from build123d import *

# Parameters (mm, degrees)
SKETCH1_R           = 75
BOSS_EXTRUDE1_DEPTH = 6.35
SKETCH2_W           = 18
SKETCH2_H           = 12
CUT_EXTRUDE1_DEPTH  = 144.69092772
CIRPATTERN1_COUNT   = 20


with BuildPart() as part:
    # Sketch1 → Boss-Extrude1 (new body)
    with BuildSketch(Plane.XY):
        with BuildLine():
            Line((-85.524663655, 39.880805624), (-96.4003571, 44.952224764))
            ThreePointArc((-96.4003571, 44.952224764), (-9.270409947, 105.961270564), (87.129947152, 61.0090458))
            Line((87.129947152, 61.0090458), (77.300122621, 54.126128564))
            ThreePointArc((77.300122621, 54.126128564), (8.224541034, -94.006934187), (-85.524663655, 39.880805624))
        make_face()
        with Locations(Location((0, 0, 0), (0, 0, 180))):
            Circle(SKETCH1_R, mode=Mode.SUBTRACT)
    boss_extrude1 = extrude(amount=BOSS_EXTRUDE1_DEPTH)

    # Mirror1: Boss-Extrude1 across plane
    add(boss_extrude1.mirror(Plane.ZX))

    # Sketch2 → Cut-Extrude1 (cut, through all)
    with BuildSketch(Plane.XY.offset(6.35)):
        with Locations((0, 82.5)):
            Rectangle(SKETCH2_W, SKETCH2_H)
    cut_extrude1 = extrude(amount=-CUT_EXTRUDE1_DEPTH, mode=Mode.SUBTRACT)

    # CirPattern1: Cut-Extrude1 ×20 about axis
    cirpattern1_axis = Axis((0, 0, 0), (0, 0, 1))
    for i in range(1, CIRPATTERN1_COUNT):
        add(cut_extrude1.rotate(cirpattern1_axis, i * 360 / CIRPATTERN1_COUNT), mode=Mode.SUBTRACT)


solid = part.part
Check sheet for the modelled part. Datum: model origin and axes. Units: mm. Round coordinates to 2 decimals unless told otherwise and drop trailing zeros. Order: outer loops, then holes, each group sorted by start corner. A loop starts at its lowest first (then second) coordinate and runs counter-clockwise, first axis right, second up.
(1) Cross-section at B-B, the plane y = 0. Enter the section's corners in (x, z).
(2) Go/stop test with flat-tipped pins: P1, Ø2, axis at y = -80, z = 5, coming from the -X side; P2, Ø3, axis at y = -3, z = 2, coming from the +X side; P3, Ø1.5, axis at x = -59.5, z = 1, coming from the -Y side. Record where each tip stops, or that it passes through.
(3) Cross-section at A-A, the plane x = 0. Enter the section's corners in (y, z).
(4) Cross-section at C-C, the plane z = 1.25. State how many separate pieces and enclosed holes the cut face has, and give its area (3 significant figures).
(5) Scan lines: probe 1 along Y at (x, z) = (0, 1.5); probe 2 along X at (y, z) = (-81, 3.5); probe 3 along Y at (x, z) = (-48, 2.75). Record each from-to range of solid material in increasing order.
Check sheet entries:
1. outline: (-94.37, 0) - (-88.5, 0) - (-88.5, 6.35) - (-94.37, 6.35) - close; (-76.5, 0) - (-75, 0) - (-75, 6.35) - (-76.5, 6.35) - close; (75, 0) - (76.5, 0) - (76.5, 6.35) - (75, 6.35) - close; (88.5, 0) - (94.37, 0) - (94.37, 6.35) - (88.5, 6.35) - close
2. P1: stops at x = -71.22
2. P2: stops at x = 94.35
2. P3: stops at y = -88.67
3. outline: (-106.37, 0) - (-88.5, 0) - (-88.5, 6.35) - (-106.37, 6.35) - close; (-76.5, 0) - (-75, 0) - (-75, 6.35) - (-76.5, 6.35) - close; (75, 0) - (76.5, 0) - (76.5, 6.35) - (75, 6.35) - close; (88.5, 0) - (106.37, 0) - (106.37, 6.35) - (88.5, 6.35) - close
4. separate pieces: 1
4. enclosed holes: 21
4. area: 11,000 mm2
5. probe 1: y = -106.37 to -88.5, -76.5 to -75, 75 to 76.5, 88.5 to 106.37
5. probe 2: x = -68.94 to -35.78, -16.86 to -9, 9 to 16.86, 35.78 to 68.94
5. probe 3: y = -94.92 to -74.52, -59.69 to -57.63, 57.63 to 59.69, 74.52 to 94.92
